```python
from build123d import *

# Parameters (mm, degrees)
F0_R     = 6
F1_DEPTH = 25
F3_W     = 12
F3_H     = 47.911397
F4_DEPTH = 60.286648


with BuildPart() as f1:
    # F0 (on Front) → F1 (new body)
    with BuildSketch(Plane.XZ):
        with BuildLine():
            Line((1.585648, -66.477157), (1.585648, 19.522843))
            ThreePointArc((1.585648, 19.522843), (-23.73806, 30.404987), (-14.203826, 4.543633))
            ThreePointArc((-14.203826, 4.543633), (-11.512447, 3.302166), (-10.414352, 0.549177))
            Line((-10.414352, 0.549177), (-10.414352, -66.477157))
            Line((-10.414352, -66.477157), (1.585648, -66.477157))
        make_face()
        with Locations((-13.414352, 19.522843)):
            Circle(F0_R, mode=Mode.SUBTRACT)
    extrude(amount=F1_DEPTH)

    # F3 (on offset) → F4 (cut, through all)
    with BuildSketch(Plane.YZ.offset(-58.7)):
        with Locations((-12, 18.478541)):
            Rectangle(F3_W, F3_H)
        with BuildLine():
            Line((-6.583733, -50.475587), (-6.590202, -25.755703))
            Line((-6.590202, -25.755703), (-6.590348, -25.195473))
            ThreePointArc((-6.590348, -25.195473), (-12.919821, -19.486577), (-18.571014, -25.867622))
            Line((-18.571014, -25.867622), (-18.583732, -50.474056))
            ThreePointArc((-18.583732, -50.474056), (-12.584498, -56.477157), (-6.583733, -50.475587))
        make_face()
    extrude(amount=F4_DEPTH, mode=Mode.SUBTRACT)


solid = f1.part
```
Model file for the job. Use its own axes, mm. A direction names the side the tool comes from. Coordinates: 2 decimals unless noted, no trailing zeros. Loops run counter-clockwise (first coordinate to the right, second up) from the corner with the lowest first, then second, coordinate; pieces in that order, holes last. Notation, with made-up numbers: (-3, 85.5) - (30, 85.5) arc R27 cw to (30, 121.5) - close; hole circle Ø3 at (54.5, 9). An arc over 180 degrees is marked (long way). Answer as a JSON object with one key per item and string values. Group by question number.
(1) Cut at D-D (x = -6.5). Give the cut face in (y, z), then the cut area to 3 significant figures.
(2) Cut at B-B (x = -23.5). Give the cut face in (y, z).
(3) Two-plate mould, pull along Z, no slides. Class faces 6 (the face through (-4, -12, -5.477)), 7 (the face through (-10, -6, 14)), 8 (the face through (-4.5, -12.79, -19.48)): released by +Z, released by -Z, zero draft, split by the parting line, or undercut.
(4) Tool access for faces 1 (the face through (-10.414, -21, -32)), 2 (the face through (-4.498, -12.716, -56.476)), 3 (the face through (-10, -18, 14)), 4 (the face through (-7, 0, -4)), 5 (the face through (-7.872, -21.451, 17.225)): list every direction of +Z, -Z, +X, -X, +Y, -Y with a clear straight run to the whole face (end or side of a thin tool).
(5) Cut at C-C (z = 22.5). Give the cut face in (x, y).
(6) Flat gauge pins, fed straight in: pin 1 (1.5 mm diameter, centred on y = -19.5, z = -22, fed in from -X); pin 2 (13 mm diameter, centred on x = -6, y = -14, fed in from +Z); pin 3 (5 mm diameter, centred on x = -5.5, y = -6.5, fed in from +Z). Where does each tip first touch, or does it go through?
(7) Probe line 1 along Y through (x, z) = (-7.5, 22); line 2 along Y through (x, z) = (0.5, -27); line 3 along X through (y, z) = (-19.5, -61). List the from-to ranges inside material, lowest first.
(8) Cut at A-A (z = -2.5). Give the cut face in (x, y).
Geometry says:
{
 "1": {"outline": "(-25, -66.48) - (0, -66.48) - (0, 32.83) - (-6, 32.83) - (-6, -5.48) - (-18, -5.48) - (-18, 32.83) - (-25, 32.83) - close; hole (-18.58, -50.47) arc R6 ccw to (-6.58, -50.48) - (-6.59, -25.76) - (-6.59, -25.2) arc R6 ccw (long way) to (-18.57, -25.87) - close", "area": "1,610 mm^2"},
 "2": {"outline": "(-25, 8.42) - (-18, 8.42) - (-18, 30.63) - (-25, 30.63) - close; (-6, 8.42) - (0, 8.42) - (0, 30.63) - (-6, 30.63) - close"},
 "3": {"face 6": "released by +Z", "face 7": "zero draft", "face 8": "undercut"},
 "4": {"face 1": "-Z, -X, +Y, -Y", "face 2": "+X, -X", "face 3": "+Z, +X, -X", "face 4": "+Z, -Z, +X, -X, +Y", "face 5": "+Y, -Y"},
 "5": {"outline": "(-28.12, -25) - (-18.62, -25) - (-18.62, -18) - (-28.12, -18) - close; (-28.12, -6) - (-18.62, -6) - (-18.62, 0) - (-28.12, 0) - close; (-8.21, -25) - (1.29, -25) - (1.29, -18) - (-8.21, -18) - close; (-8.21, -6) - (1.29, -6) - (1.29, 0) - (-8.21, 0) - close"},
 "6": {"pin 1": "stops at x = -10.41", "pin 2": "stops at z = 34.35", "pin 3": "stops at z = 33.49"},
 "7": {"line 1": "y = -25 to -18, -6 to 0", "line 2": "y = -25 to -18.57, -6.59 to 0", "line 3": "x = -10.41 to 1.59"},
 "8": {"outline": "(-10.41, -25) - (1.59, -25) - (1.59, -18) - (-10.41, -18) - close; (-10.41, -6) - (1.59, -6) - (1.59, 0) - (-10.41, 0) - close"}
}
